Check sheet for the drawn part. Datum: minimum x, y, z corner. Units: mm. A direction names the side the tool comes from. Round coordinates to 2 decimals unless told otherwise and drop trailing zeros. Loops run counter-clockwise (first coordinate to the right, second up) from the corner with the lowest first, then second, coordinate; pieces in that order, holes last.
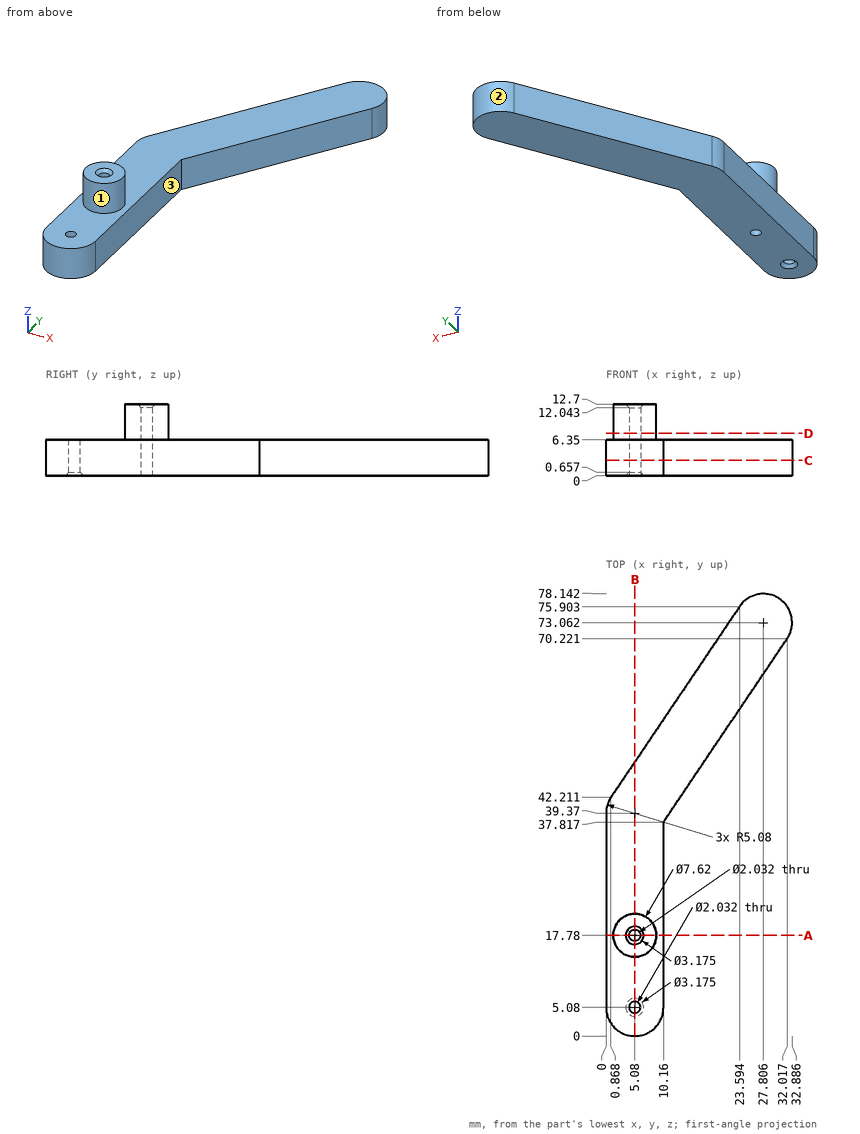
1) Scan lines: line 1 along Y through (x, z) = (5.08, 8.5) (1 decimal); line 2 along X through (y, z) = (5.08, 3.75) (1 decimal); line 3 along Y through (x, z) = (5, 3) (1 decimal). Record each from-to range of solid material in increasing order.
Report:
line 1: y = 14 to 16.8, 18.8 to 21.6
line 2: x = 0 to 4.1, 6.1 to 10.2
line 3: y = 0 to 4.1, 6.1 to 16.8, 18.8 to 48.3
2) Sectioned sample at A-A, the plane y = 17.78. Record the cut outline in (x, z).
Report:
outline: (0, 0) - (4.06, 0) - (4.06, 12.04) - (3.49, 12.7) - (1.27, 12.7) - (1.27, 6.35) - (0, 6.35) - close; (6.1, 0) - (10.16, 0) - (10.16, 6.35) - (8.89, 6.35) - (8.89, 12.7) - (6.67, 12.7) - (6.1, 12.04) - close
3) Sectioned sample at C-C, the plane z = 2.75. Record the cut outline in (x, y) (1 decimal).
Report:
outline: (0, 5.1) arc R5.1 ccw to (10.2, 5.1) - (10.2, 37.8) - (32, 70.2) arc R5.1 ccw to (23.6, 75.9) - (0.9, 42.2) arc R5.1 ccw to (0, 39.4) - close; hole circle Ø2 at (5.1, 5.1); hole circle Ø2 at (5.1, 17.8)
4) Access from +Z, -Z, +X, -X, +Y, -Y to the whole of each face (thin tool, end or side, straight path). Record for the marked faces 1, 2 and 3.
Report:
face 1: +Z
face 2: +Z, -Z
face 3: +Z, -Z, +X, -Y
5) Gauge pin test, flat ends, axial feed: pin 1 (16.5 mm diameter, centred on x = 9.5, y = 42.5, fed in from +Z); pin 2 (1.5 mm diameter, centred on y = 63.5, z = 3.5, fed in from +X); pin 3 (2.5 mm diameter, centred on x = 5.08, y = 17.78, fed in from -Z); pin 4 (1.5 mm diameter, centred on x = 8.5, z = 2, fed in from +Y) (1 decimal). Record the tip position at first contact, or that the pin passes through.
Report:
pin 1: stops at z = 6.35
pin 2: stops at x = 27.99
pin 3: stops at z = 0
pin 4: stops at y = 54.6
6) Sectioned sample at B-B, the plane x = 5.08. State how many separate pieces and enclosed holes the cut face has.
Report:
separate pieces: 3
enclosed holes: 0
7) Sectioned sample at D-D, the plane z = 7.5. Record the cut outline in (x, y).
Report:
outline: circle Ø7.62 at (5.08, 17.78); hole circle Ø2.03 at (5.08, 17.78)
